from build123d import *

# Parameters (mm, degrees)
SKETCH1_W           = 3
SKETCH1_H           = 6
BOSS_EXTRUDE1_DEPTH = 40
SKETCH2_R           = 1.75
CUT_EXTRUDE1_DEPTH  = 20
SKETCH1_3_W         = 30
SKETCH1_3_H         = 25
BOSS_EXTRUDE2_DEPTH = 10
SKETCH1_5_W         = 10
SKETCH1_5_H         = 25
BOSS_EXTRUDE3_DEPTH = 110
BOSS_EXTRUDE8_START = -110
SKETCH1_8_W         = 30
SKETCH1_8_H         = 25
SKETCH1_8_R         = 1.55
BOSS_EXTRUDE8_DEPTH = 8


with BuildPart() as part:
    # Sketch1 → Boss-Extrude1 (new body)
    with BuildSketch(Plane.XY):
        with BuildLine():
            Line((5, 17.5), (5, 11.456439237))
            ThreePointArc((5, 11.456439237), (10.458250332, 6.846531969), (12.5, 0))
            ThreePointArc((12.5, 0), (-6.846531969, -10.458250332), (-5, 11.456439237))
            Line((-5, 11.456439237), (-5, 17.5))
            Line((-5, 17.5), (-8, 17.5))
            Line((-8, 17.5), (-17.5, 17.5))
            Line((-17.5, 17.5), (-17.5, 7.5))
            Line((-17.5, 7.5), (-17.5, -17.5))
            Line((-17.5, -17.5), (17.5, -17.5))
            Line((17.5, -17.5), (17.5, 7.5))
            Line((17.5, 7.5), (17.5, 17.5))
            Line((17.5, 17.5), (8, 17.5))
            Line((8, 17.5), (5, 17.5))
        make_face()
        with Locations((-6.5, 20.5)):
            Rectangle(SKETCH1_W, SKETCH1_H)
        with Locations((6.5, 20.5)):
            Rectangle(SKETCH1_W, SKETCH1_H)
    extrude(amount=BOSS_EXTRUDE1_DEPTH)

    # Sketch2 → Cut-Extrude1 (cut)
    with BuildSketch(Plane(origin=(8, 0, 0), x_dir=(0, 0, -1), z_dir=(1, 0, 0))):
        with Locations((-25, 20.5)):
            Circle(SKETCH2_R)
        with Locations((-10, 20.5)):
            Circle(SKETCH2_R)
    extrude(amount=-CUT_EXTRUDE1_DEPTH, mode=Mode.SUBTRACT)

    # Sketch1<3> → Boss-Extrude2 (add)
    with BuildSketch(Plane.XY):
        with Locations((32.5, -5)):
            Rectangle(SKETCH1_3_W, SKETCH1_3_H)
        with Locations((-32.5, -5)):
            Rectangle(SKETCH1_3_W, SKETCH1_3_H)
    extrude(amount=BOSS_EXTRUDE2_DEPTH)

    # Sketch1<5> → Boss-Extrude3 (add)
    with BuildSketch(Plane.XY):
        with Locations((-42.5, -5)):
            Rectangle(SKETCH1_5_W, SKETCH1_5_H)
        with Locations((42.5, -5)):
            Rectangle(SKETCH1_5_W, SKETCH1_5_H)
    extrude(amount=-BOSS_EXTRUDE3_DEPTH)

    # Sketch1<8> → Boss-Extrude8 (add)
    with BuildSketch(Plane.XY.offset(BOSS_EXTRUDE8_START)):
        with Locations((62.5, -5)):
            Rectangle(SKETCH1_8_W, SKETCH1_8_H)
        with Locations((53.5, -12.5)):
            Circle(SKETCH1_8_R, mode=Mode.SUBTRACT)
        with Locations((62.5, -5)):
            Circle(SKETCH1_8_R, mode=Mode.SUBTRACT)
        with Locations((71.5, 2.5)):
            Circle(SKETCH1_8_R, mode=Mode.SUBTRACT)
        with Locations((-62.5, -5)):
            Rectangle(SKETCH1_8_W, SKETCH1_8_H)
        with Locations((-53.5, -12.5)):
            Circle(SKETCH1_8_R, mode=Mode.SUBTRACT)
        with Locations((-62.5, -5)):
            Circle(SKETCH1_8_R, mode=Mode.SUBTRACT)
        with Locations((-71.5, 2.5)):
            Circle(SKETCH1_8_R, mode=Mode.SUBTRACT)
    extrude(amount=BOSS_EXTRUDE8_DEPTH)


solid = part.part
For this review, take the finished solid that the model builds, in its own axes (mm). A direction names the side the tool comes from. Coordinates: 2 decimals unless noted, no trailing zeros. Order: outer loops, then holes, each group sorted by start corner. A loop starts at its lowest first (then second) coordinate and runs counter-clockwise, first axis right, second up. Notation, with made-up numbers: (32.5, 27.25) -> (83.5, 27.25) arc R18 ccw to (83.5, 33.25) -> close; hole circle Ø7 at (44, 18.5). An arc over 180 degrees is marked (long way). Return JSON: item names as keys, results as strings.
1. We need section B-B on z = -26.5. Write out the cut boundary in (x, y).
Answer block:
{"outline": "(-47.5, -17.5) -> (-37.5, -17.5) -> (-37.5, 7.5) -> (-47.5, 7.5) -> close; (37.5, -17.5) -> (47.5, -17.5) -> (47.5, 7.5) -> (37.5, 7.5) -> close"}
2. We need section A-A on y = 13.5. Write out the cut boundary in (x, z), and give its area (3 significant figures).
Answer block:
{"outline": "(-17.5, 0) -> (-5, 0) -> (-5, 40) -> (-17.5, 40) -> close; (5, 0) -> (17.5, 0) -> (17.5, 40) -> (5, 40) -> close", "area": "1,000 mm²"}
3. Machinability: for faces 4 (the flat face through (32, -5, 10)), 5 (the flat face through (8, -10, 0)), 6 (the flat face through (-63, -2, -102)), 7 (the flat face through (-5, 17, 20)), 8 (the flat face through (13, 17.5, 20)), which of the approach directions +Z, -Z, +X, -X, +Y, -Y give a long, thin tool a straight path to every point of the face, cutting with its end or side? Answer none if there is none.
Answer block:
{"face 4": "+Z, +X, +Y, -Y", "face 5": "-Z, +Y, -Y", "face 6": "+Z, -X, +Y, -Y", "face 7": "+Z, -Z, +Y", "face 8": "+Z, -Z, +X, +Y"}
4. We need section C-C on z = 19. Write out the cut boundary in (x, y).
Answer block:
{"outline": "(-17.5, -17.5) -> (17.5, -17.5) -> (17.5, 17.5) -> (8, 17.5) -> (8, 23.5) -> (5, 23.5) -> (5, 11.46) arc R12.5 cw (long way) to (-5, 11.46) -> (-5, 23.5) -> (-8, 23.5) -> (-8, 17.5) -> (-17.5, 17.5) -> close"}
5. For pin 1 Ø17.5 at (y, z) = (8, 19.5) entering from +X; pin 2 Ø4 at (y, z) = (20.5, 25) entering from +X; pin 3 Ø12.5 at (y, z) = (-8.5, -54.5) entering from -X; pin 4 Ø20 at (x, y) = (0, 0) entering from -Z, all flat-tipped, find the tip position at first contact; note any pin that passes through.
Answer block:
{"pin 1": "x = 17.5", "pin 2": "x = 8", "pin 3": "x = -47.5", "pin 4": "through"}
6. For line 1 (X direction, y = -6.5, z = -87); line 2 (X direction, y = 20, z = 15.5); line 3 (Y direction, x = 6.3, z = 10), list the stretches that pass through material, from the lowest coordinate up. Write a range as from..to.
Answer block:
{"line 1": "-47.5..-37.5, 37.5..47.5", "line 2": "-8..-5, 5..8", "line 3": "-17.5..-10.8, 10.8..18.75, 22.25..23.5"}
7. We need section D-D on x = 34.5. Write out the cut boundary in (y, z).
Answer block:
{"outline": "(-17.5, 0) -> (7.5, 0) -> (7.5, 10) -> (-17.5, 10) -> close"}
8. The part is to be moulded in two halves that separate along Y. For faces 1 (the cylindrical face through (6.521, 22.235, 10.228)), 2 (the flat face through (-8, 20, 20)), 3 (the flat face through (43, 7.5, -55)), say which applies: +Y half, -Y half, draft (parallel to the pull), parting line (faces both ways), or undercut.
Answer block:
{"face 1": "undercut", "face 2": "draft", "face 3": "+Y half"}
